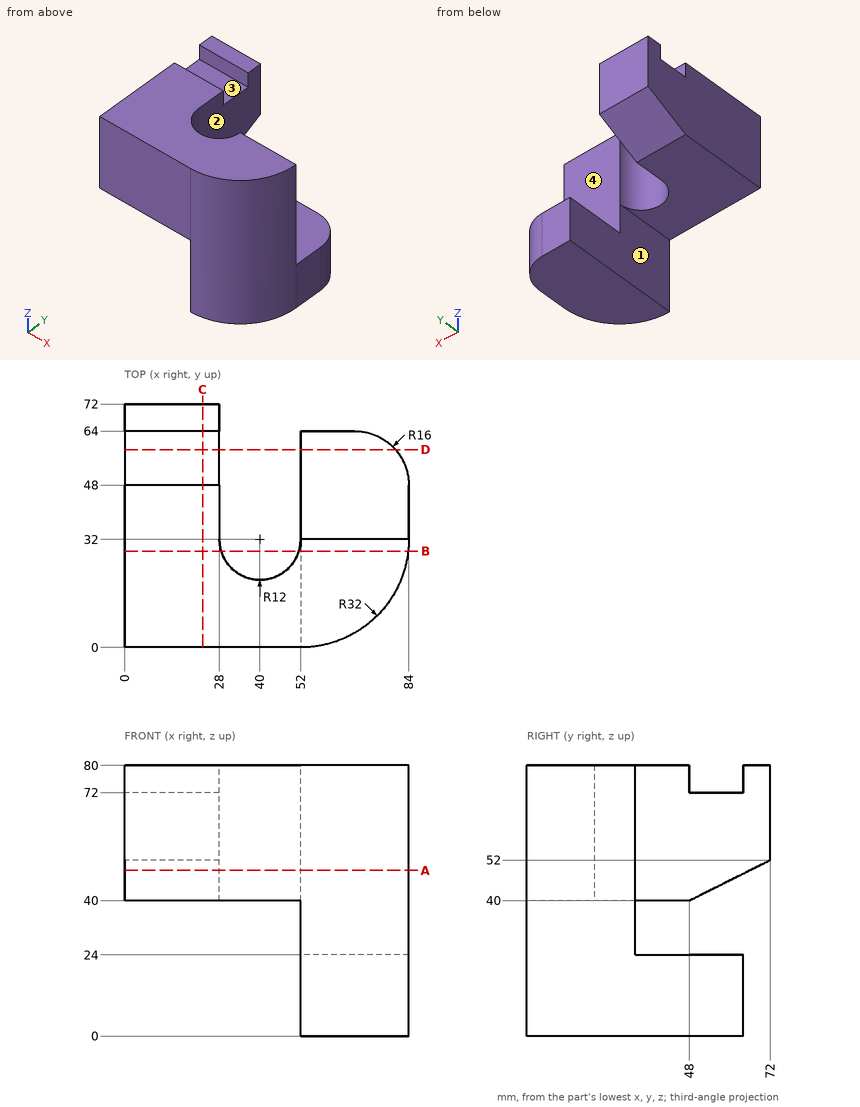
Answer from the drawing. Dimensions are ordinates in mm from the lowest x, y and z of the part. A direction names the side the tool comes from. Round coordinates to 2 decimals unless told otherwise and drop trailing zeros. Order: outer loops, then holes, each group sorted by start corner. A loop starts at its lowest first (then second) coordinate and runs counter-clockwise, first axis right, second up. Notation, with made-up numbers: (-5, 0) -> (45, 0) arc R18 cw to (45, 33) -> close; hole circle Ø11 at (42.5, 79). An arc over 180 degrees is marked (long way). Answer as CSV lines item,"result".
Q1. A cutting plane is placed at B-B on y = 28.5. Determine the outline of the cut face in (x, z), plus the area to 3 significant figures.
Computed values:
outline,"(0, 40) -> (28.52, 40) -> (28.52, 80) -> (0, 80) -> close; (51.48, 40) -> (52, 40) -> (52, 0) -> (83.81, 0) -> (83.81, 80) -> (51.48, 80) -> close"
area,"3,710 mm^2"
Q2. Consider line 1 (Z direction, x = 34, y = 14); line 2 (X direction, y = 27.5, z = 55.5); line 3 (Z direction, x = 54, y = 61). Determine where each line is inside the solid, lowest interval first. Write a range as from..to.
Computed values:
line 1,"z = 40..80"
line 2,"x = 0..28.88, 51.12..83.68"
line 3,"z = 0..24"
Q3. A cutting plane is placed at C-C on x = 23. Determine the outline of the cut face in (y, z), plus the area to 3 significant figures.
Computed values:
outline,"(0, 40) -> (48, 40) -> (72, 52) -> (72, 80) -> (64, 80) -> (64, 72) -> (48, 72) -> (48, 80) -> (0, 80) -> close"
area,"2,610 mm^2"
Q4. Which of the six approach directions +Z, -Z, +X, -X, +Y, -Y give full straight-line access (tool end or side, diameter ignored) to the marked faces 1, 2, 3 and 4?
Computed values:
face 1,"-Z, -X, +Y, -Y"
face 2,"+Z, -Z, +X, +Y"
face 3,"+Z, +X, -X"
face 4,"+Z, +X, +Y"
Q5. A cutting plane is placed at D-D on y = 58.5. Determine the outline of the cut face in (x, z).
Computed values:
outline,"(0, 45.25) -> (28, 45.25) -> (28, 72) -> (0, 72) -> close; (52, 0) -> (80.07, 0) -> (80.07, 24) -> (52, 24) -> close"
Q6. A cutting plane is placed at A-A on z = 49. Determine the outline of the cut face in (x, y), plus the area to 3 significant figures.
Computed values:
outline,"(0, 0) -> (52, 0) arc R32 ccw to (84, 32) -> (52, 32) arc R12 cw to (28, 32) -> (28, 66) -> (0, 66) -> close"
area,"3,190 mm^2"
Q7. Given pin 1 (9.5 mm diameter, centred on x = 62.5, y = 55, fed in from +Z); pin 2 (20 mm diameter, centred on y = 48, z = 60, fed in from +X); pin 3 (17.5 mm diameter, centred on x = 20.5, y = 57, fed in from +Z); pin 4 (6 mm diameter, centred on y = 21, z = 16.5, fed in from +X), each flat-ended and moving along its own axis, determine where each tip first touches the part or whether it passes through.
Computed values:
pin 1,"stops at z = 24"
pin 2,"stops at x = 28"
pin 3,"stops at z = 80"
pin 4,"stops at x = 82.98"
